Input: part model. Units: mm. Frame: model coordinates. Give positions to 0.01 mm unless a question says otherwise; leave off trailing zeros. Loops run counter-clockwise (first coordinate to the right, second up) from the corner with the lowest first, then second, coordinate; pieces in that order, holes last. Notation, with made-up numbers: M 31,-0.5 L 41,-0.5 A34 ccw 41,31.5 Z; hole C 5.5,30.5 d11. An arc over 180 degrees is marked long. Answer as a JSON object with one key per item and string values. Group by question number.
1) Section query A-A on x = -17. Return loops of the section in (y, z) (3 decimals), plus the area to 3 significant figures.
2) Ray query, L1, parallel to Y at x = 2.5, z = 1.5; L2, parallel to Y at x = 1.5, z = 1; L3, parallel to X at y = -10.5, z = 1.5. Return the intervals inside material, ascending.
3) Section query C-C on z = 0.3. Count the separate pieces of the cut face and the enclosed holes in it, plus the area to 3 significant figures.
4) First-contact query: P1, Ø1, axis at x = 22.5, z = 1, coming from the +Y side. Flat tip, straight axial feed; report the tip coordinate or a pass-through.
5) Section query B-B on y = -33. Return loops of the section in (x, z), plus the area to 3 significant figures.
6) Section query D-D on x = 2. Return loops of the section in (y, z), plus the area to 3 significant figures.
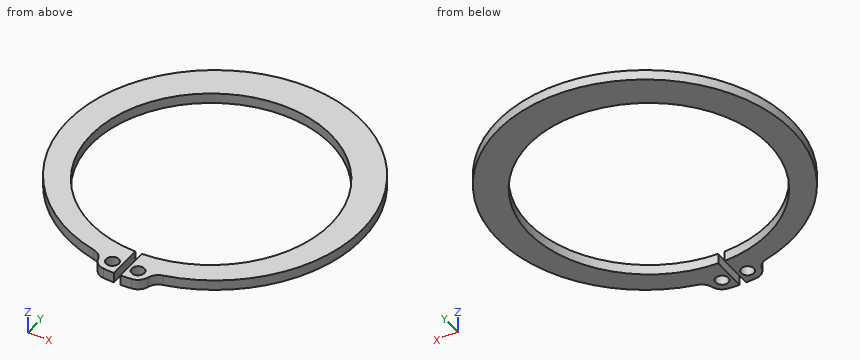
Autodesk Inventor part; units mm, degrees
ref_plane "YZ Plane" through (0, 0, 0) normal (1, 0, 0) x (0, 1, 0)
ref_plane "XZ Plane" through (0, 0, 0) normal (0, 1, 0) x (-1, 0, 0)
ref_plane "XY Plane" through (0, 0, 0) normal (0, 0, 1) x (1, 0, 0)
sketch "Skizze1" plane through (0, 0, 0) normal (0, 0, 1) x (1, 0, 0)
  line L0 (-6, 0) -> (6, 0) construction
  arc A0 (0.625, -48.4917) -> (-0.625, -48.4917) centre (0, -25) ccw
  line L1 (0, 23.3134) -> (0, -61.6825)
  line L2 (-34.59, 0) -> (46.12, 0)
  line L3 (-0.625, -48.4917) -> (-0.625, -55.3917)
  line L4 (-0.625, -6.5402) -> (-0.625, -13.29) construction
  line L5 (-2.7947, 5.1) -> (3.6722, 5.1) construction
  arc A1 (6.7169, -51.7565) -> (-6.7169, -51.7565) centre (0, -23.725) ccw
  arc A2 (-2.724, -55.2758) -> (-0.625, -55.3917) centre (0, -25) ccw
  arc A3 (-4.8997, -53.4868) -> (-2.724, -55.2758) centre (-2.5, -52.7859) ccw
  arc A4 (-4.8997, -53.4868) -> (-6.7169, -51.7565) centre (-7.2995, -54.1877) ccw
  line L6 (0.625, -48.4917) -> (0.625, -55.3917)
  line L7 (0.625, -6.5402) -> (0.625, -13.29) construction
  arc A5 (0.625, -55.3917) -> (2.724, -55.2758) centre (0, -25) ccw
  arc A6 (2.724, -55.2758) -> (4.8997, -53.4868) centre (2.5, -52.7859) ccw
  arc A7 (6.7169, -51.7565) -> (4.8997, -53.4868) centre (7.2995, -54.1877) ccw
  circle A8 centre (-2.5, -52.7859) radius 1.25
  circle A9 centre (2.5, -52.7859) radius 1.25
  dimension "d0" = 47
  dimension "d1" = 6.9
  dimension "d6" = 0.625
  dimension "d7" = 5.1
  dimension "d8" = 1.275
  dimension "d9" = 2.5
  dimension "d10" = 2.5
  dimension "d11" = 1.875
  dimension "d12" = 2.5
  dimension "d13" = 2.5
  dimension "d14" = 25
extrude "Körper" add sketch "Skizze1" along normal blind 2
equation "\"d0\" = ND"
equation "\"d1\" = SRB2"
equation "\"d6\" = 0.25 * SD5"
equation "\"d7\" = SRB1"
equation "\"d8\" = 0.25 * SRB1"
equation "\"d9\" = SD5"
equation "\"d10\" = SD5"
equation "\"d11\" = 0.75 * SD5"
equation "\"d12\" = SD5"
equation "\"d13\" = SD5"
equation "\"d14\" = 0.5 * WD"
equation "\"d2\" = SD"
equation "\"SD\" = 2"
equation "\"SRB1\" = 5.1"
equation "\"ND\" = 47"
equation "\"SRB2\" = 6.9"
equation "\"SD5\" = 2.5"
equation "\"SD3\" = 45.8"
equation "\"WDMAX\" = 52"
properties part number "R-Ring50"
Output:
{
 "1": {"outline": "M -47.003,0 L -41.225,0 L -41.225,2 L -47.003,2 Z; M -8.775,0 L -0.447,0 L -0.447,2 L -8.775,2 Z", "area": "28.2 mm^2"},
 "2": {"L1": "y = -55.3 to -54.04, -51.54 to -48.37, -1.63 to 4.99", "L2": "y = -55.36 to -53.54, -52.04 to -48.45, -1.55 to 5.06", "L3": "x = -25.61 to -18.49, 18.49 to 25.61"},
 "3": {"separate pieces": "1", "enclosed holes": "2", "area": "884 mm^2"},
 "4": {"P1": "stops at y = -5.1"},
 "5": {"outline": "M -27.29,0 L -22.1,0 L -22.1,2 L -27.29,2 Z; M 22.1,0 L 27.29,0 L 27.29,2 L 22.1,2 Z", "area": "20.8 mm^2"},
 "6": {"outline": "M -55.33,0 L -53.93,0 L -53.93,2 L -55.33,2 Z; M -51.64,0 L -48.41,0 L -48.41,2 L -51.64,2 Z; M -1.59,0 L 5.03,0 L 5.03,2 L -1.59,2 Z", "area": "22.5 mm^2"}
}
